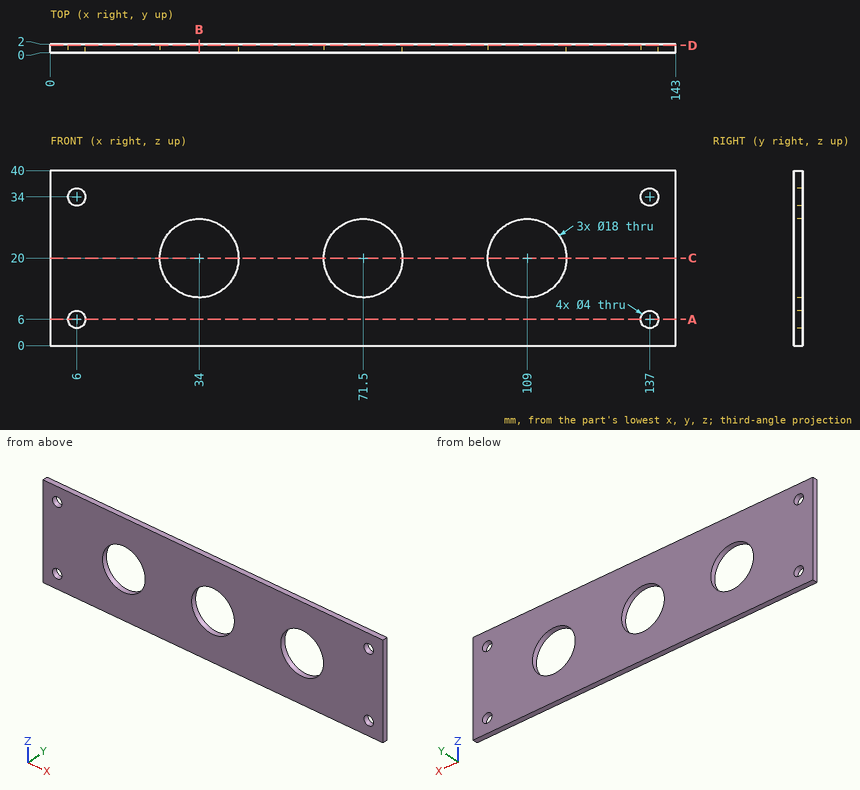
Here's the drawing with two shaded views (mm, measured from the low corner). I have some questions. Round coordinates to 2 decimals unless told otherwise and drop trailing zeros. Loops run counter-clockwise (first coordinate to the right, second up) from the corner with the lowest first, then second, coordinate; pieces in that order, holes last. Notation, with made-up numbers: (64.25, 66) -> (116.25, 66) arc R26 cw to (116.25, 97) -> close; hole circle Ø7 at (2.5, -0.75). An arc over 180 degrees is marked (long way). Answer as CSV lines item,"result". Start each with the question number.
1. I'm going to push a flat-ended pin straight in: P1, Ø1, axis at y = 1.5, z = 25, coming from the -X side. Where does the tip first touch, or does it pass through?
2. Imagine slicing it at A-A on z = 6. Write out the boundary of the cut face in (x, y), plus the area to 3 significant figures.
3. Imagine slicing it at D-D on y = 1.7. Write out the boundary of the cut face in (x, z).
4. I need wall thicknesses on probe 1 along Z at (x, y) = (137, 0.55); probe 2 along X at (y, z) = (0.5, 6); probe 3 along X at (y, z) = (0.7, 20). Which ranges of each line are inside material? Lowest first, please. Write a range as from..to.
5. Imagine slicing it at B-B on x = 34. Write out the boundary of the cut face in (y, z), plus the area to 3 significant figures.
6. Imagine slicing it at C-C on z = 20. Write out the boundary of the cut face in (x, y).
Solution:
1,P1,"x = 0"
2,outline,"(0, 0) -> (4, 0) -> (4, 2) -> (0, 2) -> close; (8, 0) -> (135, 0) -> (135, 2) -> (8, 2) -> close; (139, 0) -> (143, 0) -> (143, 2) -> (139, 2) -> close"
2,area,"270 mm²"
3,outline,"(0, 0) -> (143, 0) -> (143, 40) -> (0, 40) -> close; hole circle Ø4 at (6, 6); hole circle Ø4 at (6, 34); hole circle Ø18 at (34, 20); hole circle Ø18 at (71.5, 20); hole circle Ø18 at (109, 20); hole circle Ø4 at (137, 6); hole circle Ø4 at (137, 34)"
4,probe 1,"0..4, 8..32, 36..40"
4,probe 2,"0..4, 8..135, 139..143"
4,probe 3,"0..25, 43..62.5, 80.5..100, 118..143"
5,outline,"(0, 0) -> (2, 0) -> (2, 11) -> (0, 11) -> close; (0, 29) -> (2, 29) -> (2, 40) -> (0, 40) -> close"
5,area,"44.0 mm²"
6,outline,"(0, 0) -> (25, 0) -> (25, 2) -> (0, 2) -> close; (43, 0) -> (62.5, 0) -> (62.5, 2) -> (43, 2) -> close; (80.5, 0) -> (100, 0) -> (100, 2) -> (80.5, 2) -> close; (118, 0) -> (143, 0) -> (143, 2) -> (118, 2) -> close"
